from build123d import *

# Parameters (mm, degrees)
SKETCH1_R           = 1.5
BOSS_EXTRUDE1_DEPTH = 3


with BuildPart() as part:
    # Sketch1 → Boss-Extrude1 (new body)
    with BuildSketch(Plane(origin=(0, 0, 0), x_dir=(1, 0, 0), z_dir=(0, 1, 0))):
        with BuildLine():
            Line((0, 0), (-50, 0))
            ThreePointArc((-50, 0), (-60, 10), (-50, 20))
            Line((-50, 20), (0, 20))
            ThreePointArc((0, 20), (10, 10), (0, 0))
        make_face()
        with Locations((0, 10)):
            Circle(SKETCH1_R, mode=Mode.SUBTRACT)
        with Locations((0, 17)):
            Circle(SKETCH1_R, mode=Mode.SUBTRACT)
        with Locations((0, 3)):
            Circle(SKETCH1_R, mode=Mode.SUBTRACT)
        with Locations((7, 10)):
            Circle(SKETCH1_R, mode=Mode.SUBTRACT)
        with Locations((-7, 10)):
            Circle(SKETCH1_R, mode=Mode.SUBTRACT)
        with Locations((-50, 10)):
            Circle(SKETCH1_R, mode=Mode.SUBTRACT)
    extrude(amount=BOSS_EXTRUDE1_DEPTH)


solid = part.part
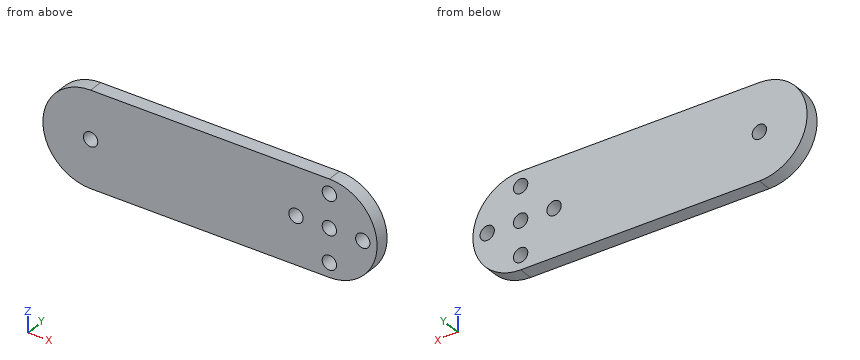
Read the model definition and answer for the solid it produces. Units are mm, in the model's axes. Coordinates: 2 decimals unless noted, no trailing zeros. Write each loop counter-clockwise with the first axis right and the second up, starting at its lowest first coordinate (ties: lowest second). Pieces come first, ordered by that corner, then holes. Notation, with made-up numbers: (-13.5, 75) - (-9.5, 75) arc R23 cw to (-9.5, 84) - close; hole circle Ø1 at (4, 41.25). An arc over 180 degrees is marked (long way). One line per question, with ' | ' between items.
Q1. Find section B-B, the plane x = -7. Write down the section's boundary in (y, z).
Result set:
outline: (0, -20) - (3, -20) - (3, -11.5) - (0, -11.5) - close; (0, -8.5) - (3, -8.5) - (3, 0) - (0, 0) - close
Q2. Find section D-D, the plane x = 7. Write down the section's boundary in (y, z), plus the area to 3 significant figures.
Result set:
outline: (0, -17.14) - (3, -17.14) - (3, -11.5) - (0, -11.5) - close; (0, -8.5) - (3, -8.5) - (3, -2.86) - (0, -2.86) - close | area: 33.8 mm^2
Q3. Each of these flat-tipped pins is pushed along its axis until it touches: P1, Ø1.5, axis at y = 1, z = -3, coming from the -X side; P2, Ø3.5, axis at x = 0, z = -17, coming from the -Y side. Where does it stop, or does it pass through?
Result set:
P1: x = -57.81 | P2: y = 0
Q4. Find section A-A, the plane y = 2.5. Write down the section's boundary in (x, z), plus the area to 3 significant figures.
Result set:
outline: (-50, -20) - (0, -20) arc R10 ccw to (0, 0) - (-50, 0) arc R10 ccw to start; hole circle Ø3 at (-50, -10); hole circle Ø3 at (-7, -10); hole circle Ø3 at (0, -17); hole circle Ø3 at (0, -10); hole circle Ø3 at (0, -3); hole circle Ø3 at (7, -10) | area: 1,270 mm^2
Q5. Consider L1, parallel to X at y = 2.2, z = -10; L2, parallel to Z at x = -7, y = 1.35; L3, parallel to Z at x = -7.5, y = 1.55. Determine where each line is inside the solid, lowest interval first. Write a range as [from, to].
Result set:
L1: [-60, -51.5], [-48.5, -8.5], [-5.5, -1.5], [1.5, 5.5], [8.5, 10] | L2: [-20, -11.5], [-8.5, 0] | L3: [-20, -11.41], [-8.59, 0]
Q6. Find section C-C, the plane z = -10. Write down the section's boundary in (x, y), plus the area to 3 significant figures.
Result set:
outline: (-60, 0) - (-51.5, 0) - (-51.5, 3) - (-60, 3) - close; (-48.5, 0) - (-8.5, 0) - (-8.5, 3) - (-48.5, 3) - close; (-5.5, 0) - (-1.5, 0) - (-1.5, 3) - (-5.5, 3) - close; (1.5, 0) - (5.5, 0) - (5.5, 3) - (1.5, 3) - close; (8.5, 0) - (10, 0) - (10, 3) - (8.5, 3) - close | area: 174 mm^2
